Work out the finished part from the listing and answer in its coordinate system (mm). A direction names the side the tool comes from. Coordinates: 2 decimals unless noted, no trailing zeros. Loops run counter-clockwise (first coordinate to the right, second up) from the corner with the lowest first, then second, coordinate; pieces in that order, holes last. Notation, with made-up numbers: (-40, -20.5) -> (3, -20.5) arc R27 cw to (3, 17.5) -> close; hole circle Ø10 at (8, 42). An arc over 180 degrees is marked (long way). Use a Markdown table: item, result.
from build123d import *

# Parameters (mm, degrees)
F1_DEPTH = 25.4
F2_W     = 130.175
F2_H     = 4.572
F3_DEPTH = 25.401
F5_DEPTH = 8.89
F6_R     = 12.7


with BuildPart() as f1:
    # F0 (on Top) → F1 (new body)
    with BuildSketch(Plane.XY):
        with BuildLine():
            Line((69.270322, 31.75), (-69.270322, 31.75))
            ThreePointArc((-69.270322, 31.75), (-76.2, 0), (-69.270322, -31.75))
            Line((-69.270322, -31.75), (69.270322, -31.75))
            ThreePointArc((69.270322, -31.75), (76.2, 0), (69.270322, 31.75))
        make_face()
    extrude(amount=F1_DEPTH)

    # F2 (on face) → F3 (cut, through all)
    with BuildSketch(Plane(origin=(0, 0, 0), x_dir=(1, 0, 0), z_dir=(0, 0, -1))):
        Rectangle(F2_W, F2_H)
    extrude(amount=-F3_DEPTH, mode=Mode.SUBTRACT)

    # F4 (on face) → F5 (cut)
    with BuildSketch(Plane(origin=(0, 0, 0), x_dir=(1, 0, 0), z_dir=(0, 0, -1))):
        Polygon((69.85, 7.62), (-69.85, 7.62), (-69.85, -7.62), (69.85, -7.62), (69.85, -3.116865), (69.85, 3.233135), align=None)
        with BuildLine():
            Line((76.131379, 3.233135), (69.85, 3.233135))
            Line((69.85, 3.233135), (69.85, -3.116865))
            Line((69.85, -3.116865), (76.136228, -3.116865))
            ThreePointArc((76.136228, -3.116865), (76.199978, 0.058186), (76.131379, 3.233135))
        make_face()
    extrude(amount=-F5_DEPTH, mode=Mode.SUBTRACT)

    # F6
    f6_edges = [f1.edges().sort_by_distance(p)[0] for p in [
        (69.270322, -31.75, 12.7),
        (69.270322, 31.75, 12.7),
        (-69.270322, -31.75, 12.7),
        (-69.270322, 31.75, 12.7),
    ]]
    fillet(f6_edges, radius=F6_R)


solid = f1.part
Q1. Section A-A on x = -57 is taken. Determine the outline of the cut face in (y, z), and give its area (3 significant figures).
Solved:
| item | result |
|---|---|
| outline | (-31.75, 0) -> (-7.62, 0) -> (-7.62, 8.89) -> (-2.29, 8.89) -> (-2.29, 25.4) -> (-31.75, 25.4) -> close; (2.29, 8.89) -> (7.62, 8.89) -> (7.62, 0) -> (31.75, 0) -> (31.75, 25.4) -> (2.29, 25.4) -> close |
| area | 1,400 mm² |
Q2. Determine the mould class of faces 5 (the flat face through (-1, 15, 0)), 6 (the flat face through (2, -3, 8.89)), 7 (the cylindrical face through (-76.2, 0.3, 12.5)) for opening direction Y: pulls with the +Y half, pulls with the -Y half, needs draft (parallel to the pull), parting line crosses it, or undercut.
Solved:
| item | result |
|---|---|
| face 5 | needs draft |
| face 6 | undercut |
| face 7 | parting line crosses it |
Q3. Given pin 1 Ø1.4 at (y, z) = (1, 17) entering from -X; pin 2 Ø2.5 at (y, z) = (0.5, 5.5) entering from +X; pin 3 Ø4.5 at (x, y) = (-8.5, -3.5) entering from -Z, each flat-ended and moving along its own axis, determine where each tip first touches the part or whether it passes through.
Solved:
| item | result |
|---|---|
| pin 1 | x = -76.2 |
| pin 2 | x = -69.85 |
| pin 3 | z = 8.89 |
Q4. Section C-C on z = 4 is taken. Determine the outline of the cut face in (x, y), and give its area (3 significant figures).
Solved:
| item | result |
|---|---|
| outline | (-72.69, -22.86) arc R12.7 ccw to (-60.58, -31.75) -> (60.58, -31.75) arc R12.7 ccw to (72.69, -22.86) arc R76.2 ccw to (76.13, -3.23) -> (69.85, -3.23) -> (69.85, -7.62) -> (-69.85, -7.62) -> (-69.85, 7.62) -> (69.85, 7.62) -> (69.85, 3.12) -> (76.14, 3.12) arc R76.2 ccw to (72.69, 22.86) arc R12.7 ccw to (60.58, 31.75) -> (-60.58, 31.75) arc R12.7 ccw to (-72.69, 22.86) arc R76.2 ccw to start |
| area | 7,160 mm² |
Q5. Section B-B on z = 22 is taken. Determine the outline of the cut face in (x, y), and give its area (3 significant figures).
Solved:
| item | result |
|---|---|
| outline | (-72.69, -22.86) arc R12.7 ccw to (-60.58, -31.75) -> (60.58, -31.75) arc R12.7 ccw to (72.69, -22.86) arc R76.2 ccw to (72.69, 22.86) arc R12.7 ccw to (60.58, 31.75) -> (-60.58, 31.75) arc R12.7 ccw to (-72.69, 22.86) arc R76.2 ccw to start; hole (-65.09, -2.29) -> (65.09, -2.29) -> (65.09, 2.29) -> (-65.09, 2.29) -> close |
| area | 8,740 mm² |
Q6. Consider line 1 (Y direction, x = 8, z = 19.5); line 2 (X direction, y = 0, z = 10); line 3 (Y direction, x = 16, z = 5.5). Determine where each line is inside the solid, lowest interval first. Write a range as [from, to].
Solved:
| item | result |
|---|---|
| line 1 | [-31.75, -2.29], [2.29, 31.75] |
| line 2 | [-76.2, -65.09], [65.09, 76.2] |
| line 3 | [-31.75, -7.62], [7.62, 31.75] |
Q7. For faces 1 (the flat face through (73, 3.117, 4)), 2 (the flat face through (65.088, 0, 17)), 3 (the flat face through (-1, 7.62, 4)), 4 (the cylindrical face through (-67.998, 29.355, 12.878)), determine the directions among +Z, -Z, +X, -X, +Y, -Y from which every point of the face is accessible in a straight line to the end or side of a thin tool.
Solved:
| item | result |
|---|---|
| face 1 | -Z, +X |
| face 2 | +Z, -Z |
| face 3 | -Z |
| face 4 | +Z, -Z, -X, +Y |
Q8. Section D-D on y = -17.5 is taken. Determine the outline of the cut face in (x, z).
Solved:
| item | result |
|---|---|
| outline | (-74.16, 0) -> (74.16, 0) -> (74.16, 25.4) -> (-74.16, 25.4) -> close |
